Geometry: final body of the model. Coordinates: model frame, mm. A direction names the side the tool comes from. Coordinates: 2 decimals unless noted, no trailing zeros. Loops run counter-clockwise (first coordinate to the right, second up) from the corner with the lowest first, then second, coordinate; pieces in that order, holes last. Notation, with made-up numbers: (32.25, 35) - (78.25, 35) arc R18 ccw to (78.25, 39) - close; hole circle Ø11 at (48.5, -22.75). An arc over 180 degrees is marked (long way). Return JSON: item names as keys, results as strings.
Autodesk Inventor part; units mm, degrees
ref_plane "YZ Plane" through (0, 0, 0) normal (1, 0, 0) x (0, 1, 0)
ref_plane "XZ Plane" through (0, 0, 0) normal (0, 1, 0) x (-1, 0, 0)
ref_plane "XY Plane" through (0, 0, 0) normal (0, 0, 1) x (1, 0, 0)
sketch "Sketch1" plane through (0, 0, 0) normal (0, 0, 1) x (1, 0, 0)
  line L0 (0, 23.05) -> (0, 23.05)
  line L1 (4, 19.05) -> (4, 12.3438)
  line L2 (0, -23.05) -> (0, -23.05)
  line L3 (-4, -19.05) -> (-4, -9.6314)
  line L4 (-4, 23.05) -> (0, 23.05) construction
  line L5 (0, 23.05) -> (0, 0) construction
  line L6 (0, 0) -> (-4, 0) construction
  line L7 (-4, 0) -> (-4, 23.05) construction
  arc A0 (4, 19.05) -> (0, 23.05) centre (0, 19.05) ccw
  arc A1 (0, 23.05) -> (-4, 19.05) centre (0, 19.05) ccw
  arc A2 (-4, -19.05) -> (0, -23.05) centre (0, -19.05) ccw
  arc A3 (0, -23.05) -> (4, -19.05) centre (0, -19.05) ccw
  line L8 (-4, 7.0746) -> (4, 12.3438)
  line L9 (-4, 7.0746) -> (-4, 19.05)
  line L10 (4, 12.3438) -> (4, -14.8227)
  line L11 (-4, -9.6314) -> (4, -14.8227)
  line L12 (-4, -9.6314) -> (-4, 7.0746)
  line L13 (4, -14.8227) -> (4, -19.05)
  dimension "d0" = 4
  dimension "d6" = 38.1
extrude "Extrusion5" add sketch "Sketch1" along normal mid plane 10
extrude "Extrusion6" cut sketch "Sketch1" along normal mid plane 5 contours L1 L8 L9 A1 A0 | L13 A3 A2 L3 L11
sketch "Sketch4" plane through (0, 0, 5) normal (0, 0, 1) x (1, 0, 0)
  arc A0 (4, 19.05) -> (-4, 19.05) centre (0, 19.05) ccw
  arc A1 (-4, -19.05) -> (4, -19.05) centre (0, -19.05) ccw
  point P0 (0, 0)
hole "Hole3" at (0, -19.05, 5) at (0, 19.05, 5) direction (0, 0, -1) diameter 3.4 end through all
fillet "Fillet1" radius 2 4 edges at (4, -14.8227, 0) (4, 12.3438, 0) (-4, 7.0746, 0) (-4, -9.6314, 0)
sketch "Sketch5" plane through (0, 0, -2.5) normal (0, 0, 1) x (1, 0, 0)
  circle A0 centre (0, -19.05) radius 1.7
  arc A1 (-4, -19.05) -> (4, -19.05) centre (0, -19.05) ccw
  line L0 (4, -11.1407) -> (4, -19.05)
  arc A2 (0.9113, -12.8184) -> (4, -11.1407) centre (2, -11.1407) ccw
  line L1 (0.9113, -12.8184) -> (-3.0887, -10.2228)
  arc A3 (-4, -8.5451) -> (-3.0887, -10.2228) centre (-2, -8.5451) ccw
  line L2 (-4, -19.05) -> (-4, -8.5451)
  point P0 (0, 0)
extrude "Extrusion7" cut sketch "Sketch5" against normal through all
equation "\"d6\" = LengthK"
properties part number "F"
Item 1: Mould query, pull axis Y, two halves, no side actions, for faces 1 (the face through (-3.764, -9.487, -3.732)), 2 (the face through (0, 15, -2.5)), 3 (the face through (-0.07, -17.35, 3.73)), 4 (the face through (-1.128, 8.966, -0.035)). Classes: +Y half, -Y half, draft (parallel to the pull), parting line (faces both ways), or undercut.
Worked out:
{"face 1": "-Y half", "face 2": "draft", "face 3": "undercut", "face 4": "+Y half"}
Item 2: Section query C-C, the plane y = -12. Return loops of the section in (x, z).
Worked out:
{"outline": "(-4, 2.5) - (-0.35, 2.5) - (-0.35, -5) - (3.81, -5) - (3.81, 2.5) - (4, 2.5) - (4, 5) - (-4, 5) - close"}
Item 3: Section query A-A, the plane z = -3.75. Return loops of the section in (x, y), and give its area (3 significant figures).
Worked out:
{"outline": "(-4, -8.55) arc R2 ccw to (-3.09, -10.22) - (0.91, -12.82) arc R2 ccw to (4, -11.14) - (4, 19.05) arc R4 ccw to (-4, 19.05) - close; hole circle Ø3.4 at (0, 19.05)", "area": "263 mm^2"}
Item 4: First-contact query: pin 1 Ø1.5 at (x, z) = (-2, 2.5) entering from +Y; pin 2 Ø2.5 at (x, y) = (-0.5, -14.5) entering from -Z. Flat tips, straight axial feed; report the tip coordinate or a pass-through.
Worked out:
{"pin 1": "y = 22.85", "pin 2": "z = 2.5"}
Item 5: Ray query, probe 1 along Y at (x, z) = (0, 3.35); probe 2 along X at (y, z) = (19.05, -4); probe 3 along Z at (x, y) = (-2.75, 10.5). Return the intervals inside material, ascending. Write a range as from..to.
Worked out:
{"probe 1": "-23.05..-20.75, -17.35..17.35, 20.75..23.05", "probe 2": "-4..-1.7, 1.7..4", "probe 3": "-5..-2.5, 2.5..5"}
Item 6: Reachability of faces 5 (the face through (-3.764, -9.487, 0.035)), 6 (the face through (2.922, 10.406, -0.035)), 7 (the face through (-3.77, 6.93, -0.04)), 8 (the face through (4, 0, 0)), 9 (the face through (0, 5, -5)) from +Z, -Z, +X, -X, +Y, -Y: full face, straight path, thin tool, end or side. Return the list, or none.
Worked out:
{"face 5": "-Z, -X, -Y", "face 6": "+Y", "face 7": "-X, +Y", "face 8": "+Z, -Z, +X, +Y, -Y", "face 9": "-Z, +X, -X, +Y, -Y"}
Item 7: Section query D-D, the plane z = -2. Return loops of the section in (x, y).
Worked out:
{"outline": "(-4, -8.55) arc R2 ccw to (-3.09, -10.22) - (0.91, -12.82) arc R2 ccw to (4, -11.14) - (4, 8.63) arc R2 ccw to (0.9, 10.3) - (-3.1, 7.67) arc R2 ccw to (-4, 6) - close"}
Item 8: Section query B-B, the plane x = 0. Return loops of the section in (y, z), and give its area (3 significant figures).
Worked out:
{"outline": "(-23.05, 2.5) - (-20.75, 2.5) - (-20.75, 5) - (-23.05, 5) - close; (-17.35, 2.5) - (-12.23, 2.5) - (-12.23, -5) - (17.35, -5) - (17.35, -2.5) - (9.71, -2.5) - (9.71, 2.5) - (17.35, 2.5) - (17.35, 5) - (-17.35, 5) - close; (20.75, -5) - (23.05, -5) - (23.05, -2.5) - (20.75, -2.5) - close; (20.75, 2.5) - (23.05, 2.5) - (23.05, 5) - (20.75, 5) - close", "area": "288 mm^2"}
